The listing builds one solid part. Answer for the finished solid, in the listing's coordinates (mm). A direction names the side the tool comes from. Round coordinates to 2 decimals unless told otherwise and drop trailing zeros. Write each loop counter-clockwise with the first axis right and the second up, starting at its lowest first coordinate (ties: lowest second). Pieces come first, ordered by that corner, then holes. Notation, with made-up numbers: (76, 74.25) - (127, 74.25) arc R20 ccw to (127, 91.25) - close; hole circle Ø7 at (74.5, 13.5). An arc over 180 degrees is marked (long way). Return JSON: item names as keys, results as strings. Group by question number.
(1) Section B-B, the plane z = 0 is taken. Write down the section's boundary in (x, y).
(2) Each of these flat-tipped pins is pushed along its axis until it touches: pin 1 (8 mm diameter, centred on x = 3, z = 0.5, fed in from +Y); pin 2 (2 mm diameter, centred on y = 0, z = -6.5, fed in from +X). Where does it stop, or does it pass through?
(3) Which of the six approach directions +Z, -Z, +X, -X, +Y, -Y give full straight-line access (tool end or side, diameter ignored) to faces 4 (the flat face through (-8, 0, -11)), 5 (the cylindrical face through (3.9, 1.1, 12.4)), 6 (the flat face through (0, -3.3, 0))?
(4) Determine the mould class of faces 1 (the flat face through (0, 0.4, 0)), 2 (the cylindrical face through (0.66, 0.838, -14.985)), 3 (the flat face through (5.3, -1.2, 5.3)) for opening direction Z: +Z half, -Z half, draft (parallel to the pull), parting line (faces both ways), or undercut.
(5) Section A-A, the plane x = 0 is taken. Write down the section's boundary in (y, z).
(6) Find the intervals of material crossed by line 1 along X through (y, z) = (0.8, -0.25); line 2 along Y through (x, z) = (5.75, -1); line 3 along Y through (x, z) = (11.75, 0), in increasing order. Write a range as [from, to].
```python
from build123d import *

# Parameters (mm, degrees)
SKETCH_1_R          = 15
EXTRUDE_1_DEPTH     = 1.7
SKETCH_2_R          = 13.403606185
EXTRUDE_2_DEPTH     = 1.2
FILLET_1_R          = 1
SKETCH_4_R          = 7.153275754
EXTRUDE_3_DEPTH     = 2.1
SKETCH_6_R          = 12.998633497
CUT_EXTRUDE_4_DEPTH = 1.3


with BuildPart() as part:
    # Эскиз1 → Бобышка-Вытянуть1 (new body)
    with BuildSketch(Plane(origin=(0, 0, 0), x_dir=(1, 0, 0), z_dir=(0, 1, 0))):
        with Locations(Location((0, 0, 0), (0, 0, 270))):
            Circle(SKETCH_1_R)
    extrude(amount=EXTRUDE_1_DEPTH)

    # Эскиз2 → Бобышка-Вытянуть2 (add)
    with BuildSketch(Plane.XZ):
        with Locations(Location((0, 0, 0), (0, 0, 90))):
            Circle(SKETCH_2_R)
    extrude(amount=EXTRUDE_2_DEPTH)

    # Скругление1
    fillet_1_edges = [part.edges().sort_by_distance(p)[0] for p in [
        (0, -1.2, -13.403606185),
    ]]
    fillet(fillet_1_edges, radius=FILLET_1_R)

    # Эскиз4 → Бобышка-Вытянуть3 (add)
    with BuildSketch(Plane.XZ.offset(1.2)):
        with Locations(Location((0, 0, 0), (0, 0, 270))):
            Circle(SKETCH_4_R)
    extrude(amount=EXTRUDE_3_DEPTH)

    # Эскиз6 → Вырез-Вытянуть4 (cut)
    with BuildSketch(Plane(origin=(0, 1.7, 0), x_dir=(1, 0, 0), z_dir=(0, 1, 0))):
        with Locations(Location((0, 0, 0), (0, 0, 270))):
            Circle(SKETCH_6_R)
    extrude(amount=-CUT_EXTRUDE_4_DEPTH, mode=Mode.SUBTRACT)


solid = part.part
```
Working result:
{
 "1": {"outline": "(-15, 0) - (-13.4, 0) - (-13.4, -0.2) arc R1 ccw to (-12.4, -1.2) - (-7.15, -1.2) - (-7.15, -3.3) - (7.15, -3.3) - (7.15, -1.2) - (12.4, -1.2) arc R1 ccw to (13.4, -0.2) - (13.4, 0) - (15, 0) - (15, 1.7) - (13, 1.7) - (13, 0.4) - (-13, 0.4) - (-13, 1.7) - (-15, 1.7) - close"},
 "2": {"pin 1": "stops at y = 0.4", "pin 2": "stops at x = 13.96"},
 "3": {"face 4": "-Y", "face 5": "+Y", "face 6": "+Z, -Z, +X, -X, -Y"},
 "4": {"face 1": "undercut", "face 2": "parting line", "face 3": "draft"},
 "5": {"outline": "(-3.3, -7.15) - (-1.2, -7.15) - (-1.2, -12.4) arc R1 ccw to (-0.2, -13.4) - (0, -13.4) - (0, -15) - (1.7, -15) - (1.7, -13) - (0.4, -13) - (0.4, 13) - (1.7, 13) - (1.7, 15) - (0, 15) - (0, 13.4) - (-0.2, 13.4) arc R1 ccw to (-1.2, 12.4) - (-1.2, 7.15) - (-3.3, 7.15) - close"},
 "6": {"line 1": "x = [-15, -13], [13, 15]", "line 2": "y = [-3.3, 0.4]", "line 3": "y = [-1.2, 0.4]"}
}
